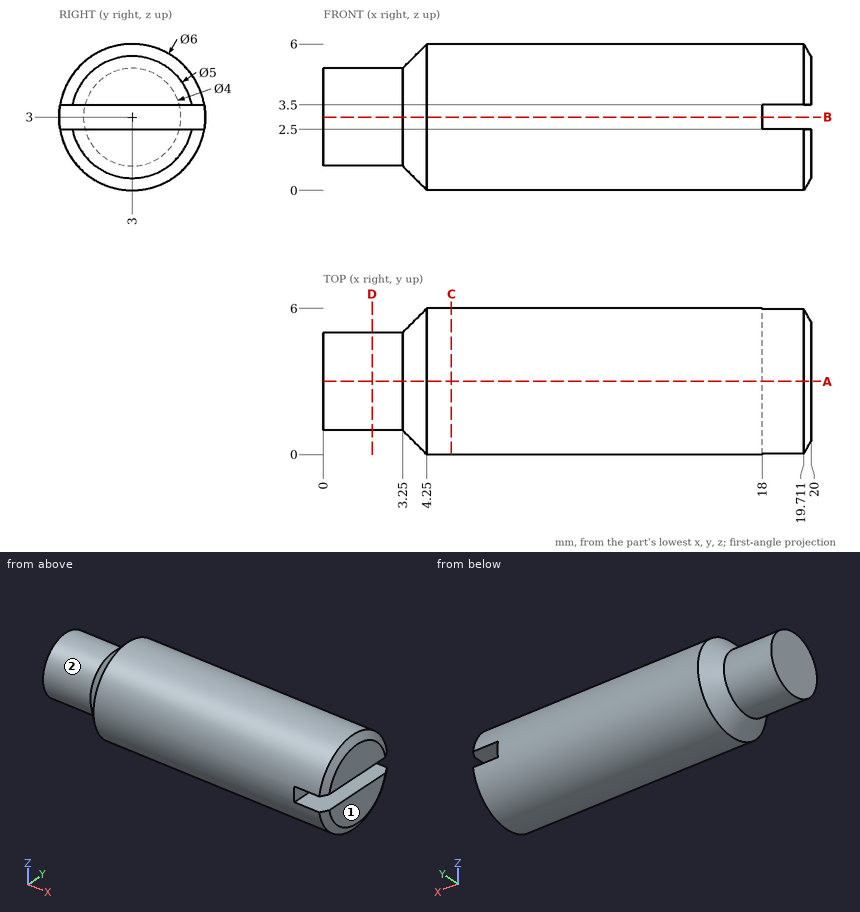
Here's the drawing with two shaded views (mm, measured from the low corner). I have some questions. A direction names the side the tool comes from. Round coordinates to 2 decimals unless told otherwise and drop trailing zeros. Loops run counter-clockwise (first coordinate to the right, second up) from the corner with the lowest first, then second, coordinate; pieces in that order, holes last. Notation, with made-up numbers: M 16.25,87 L 73.25,87 A18 ccw 73.25,104 Z; hole C -13.75,57.5 d1. An arc over 180 degrees is marked long. Answer as CSV lines item,"result".
1) Imagine slicing it at B-B on z = 3. List the corners of the cut face in (x, y) for me, and give its area (4 significant figures).
From the geometry:
outline,"M 0,1 L 3.25,1 L 4.25,0 L 18,0 L 18,6 L 4.25,6 L 3.25,5 L 0,5 Z"
area,"100.5 mm^2"
2) For pin 1 Ø3 at (y, z) = (5, 5) entering from -X; pin 2 Ø0.5 at (y, z) = (3, 3) entering from +X; pin 3 Ø1.6 at (x, y) = (18.5, 4) entering from -Z, each with a flat end and sliding along its axis, tell me the tip position at first contact or that it passes through.
From the geometry:
pin 1,"x = 0"
pin 2,"x = 18"
pin 3,"z = 0.01"
3) Imagine slicing it at C-C on x = 5.25. List the corners of the cut face in (y, z) for me, and give its area (3 significant figures).
From the geometry:
outline,"C 3,3 d6"
area,"28.3 mm^2"
4) Imagine slicing it at A-A on y = 3. List the corners of the cut face in (x, z) for me.
From the geometry:
outline,"M 0,1 L 3.25,1 L 4.25,0 L 19.71,0 L 20,0.5 L 20,2.5 L 18,2.5 L 18,3.5 L 20,3.5 L 20,5.5 L 19.71,6 L 4.25,6 L 3.25,5 L 0,5 Z"
5) Which directions (+Z, -Z, +X, -X, +Y, -Y) give clear straight access to the entire face, cutting with the end or side of a thin tool? Please do the marked faces 1 and 2.
From the geometry:
face 1,"+Z, -Z, +X, +Y, -Y"
face 2,"-X"
6) If I drill on probe 1 along X at (y, z) = (1.95, 3.15); probe 2 along Y at (x, z) = (4.75, 2.1); probe 3 along Z at (x, y) = (15, 3.5), over which ranges is the centre line in solid material (lowest first)?
From the geometry:
probe 1,"0 to 18"
probe 2,"0.14 to 5.86"
probe 3,"0.04 to 5.96"
7) Imagine slicing it at D-D on x = 2. List the corners of the cut face in (y, z) for me.
From the geometry:
outline,"C 3,3 d4"
